For this review, take the finished solid that the model builds, in its own axes (mm). A direction names the side the tool comes from. Round coordinates to 2 decimals unless told otherwise and drop trailing zeros. Order: outer loops, then holes, each group sorted by start corner. A loop starts at its lowest first (then second) coordinate and runs counter-clockwise, first axis right, second up. Notation, with made-up numbers: (50, -31) - (95, -31) arc R8 cw to (95, -21) - close; hole circle Ø3 at (32.5, -19.75). An arc over 180 degrees is marked (long way). One line per question, with ' | ' between items.
```python
from build123d import *

# Parameters (mm, degrees)
SKETCH2_R           = 40
BOSS_EXTRUDE1_DEPTH = 320
SKETCH3_R           = 30
CUT_EXTRUDE1_DEPTH  = 300
CUT_EXTRUDE2_REACH  = 326.962
SKETCH4_R           = 22.5
BOSS_EXTRUDE2_START = 80
SKETCH5_R           = 40
BOSS_EXTRUDE2_DEPTH = 80
SKETCH6_W           = 40
SKETCH6_H           = 78
CUT_EXTRUDE3_DEPTH  = 5
SKETCH7_R           = 15
CUT_EXTRUDE4_DEPTH  = 332.096662623
FILLET2_R           = 5
FILLET3_R           = 2


with BuildPart() as part:
    # Sketch2 → Boss-Extrude1 (new body)
    with BuildSketch(Plane.XY):
        Circle(SKETCH2_R)
    extrude(amount=BOSS_EXTRUDE1_DEPTH)

    # Sketch3 → Cut-Extrude1 (cut)
    with BuildSketch(Plane(origin=(0, 0, 0), x_dir=(-1, 0, 0), z_dir=(0, 0, -1))):
        Circle(SKETCH3_R)
    extrude(amount=-CUT_EXTRUDE1_DEPTH, mode=Mode.SUBTRACT)

    # Sketch4 → Cut-Extrude2 (cut, up to next)
    with BuildSketch(Plane.XY.offset(320), mode=Mode.PRIVATE) as cut_extrude2_sk1:
        Circle(SKETCH4_R)
    cut_extrude2_tool1 = extrude(cut_extrude2_sk1.sketch, amount=-CUT_EXTRUDE2_REACH, mode=Mode.PRIVATE) & part.part
    add(cut_extrude2_tool1.solids().sort_by_distance((0, 0, 320))[0], mode=Mode.SUBTRACT)

    # Sketch5 → Boss-Extrude2 (add)
    with BuildSketch(Plane(origin=(0, 0, 0), x_dir=(-1, 0, 0), z_dir=(0, 0, -1)).offset(BOSS_EXTRUDE2_START)):
        Circle(SKETCH5_R)
    extrude(amount=-BOSS_EXTRUDE2_DEPTH)

    # Sketch6 → Cut-Extrude3 (cut)
    with BuildSketch(Plane(origin=(0, 40, 0), x_dir=(1, 0, 0), z_dir=(0, 1, 0))):
        with Locations((0, 41)):
            Rectangle(SKETCH6_W, SKETCH6_H)
    cut_extrude3 = extrude(amount=-CUT_EXTRUDE3_DEPTH, mode=Mode.SUBTRACT)

    # Mirror1: Cut-Extrude3 across plane
    add(cut_extrude3.mirror(Plane.ZX), mode=Mode.SUBTRACT)

    # Sketch7 → Cut-Extrude4 (cut, through all)
    with BuildSketch(Plane(origin=(0, 35, 0), x_dir=(1, 0, 0), z_dir=(0, 1, 0))):
        with Locations(Location((0, 45, 0), (0, 0, 270))):
            Circle(SKETCH7_R)
    extrude(amount=-CUT_EXTRUDE4_DEPTH, mode=Mode.SUBTRACT)

    # Fillet2
    fillet2_edges = [part.edges().sort_by_distance(p)[0] for p in [
        (40, 0, -80),
        (0, 35, -80),
        (-34.457195687, 20.315060063, -80),
        (0, -35, -80),
        (-40, 0, 320),
    ]]
    fillet(fillet2_edges, radius=FILLET2_R - 0.0001)  # a hair under: the kernel refuses the full size

    # Fillet3
    fillet3_edges = [part.edges().sort_by_distance(p)[0] for p in [
        (0, -35, -60),
        (0, 35, -60),
    ]]
    fillet(fillet3_edges, radius=FILLET3_R)


solid = part.part
```
(1) We need section A-A on x = 0. State the section outline as (y, z) points, plus the area to 3 significant figures.
Output values:
outline: (-40, -2) - (-35, -2) - (-35, -28) arc R2 ccw to (-33, -30) - (33, -30) arc R2 ccw to (35, -28) - (35, -2) - (40, -2) - (40, 315) arc R5 ccw to (35, 320) - (22.5, 320) - (22.5, 300) - (30, 300) - (30, 0) - (-30, 0) - (-30, 300) - (-22.5, 300) - (-22.5, 320) - (-35, 320) arc R5 ccw to (-40, 315) - close; (-35, -75) arc R5 ccw to (-30, -80) - (30, -80) arc R5 ccw to (35, -75) - (35, -62) arc R2 ccw to (33, -60) - (-33, -60) arc R2 ccw to (-35, -62) - close | area: 10,200 mm^2
(2) Insertion check: pin 1 (6 mm diameter, centred on x = 29.5, z = 93.5, fed in from -Y); pin 2 (1.5 mm diameter, centred on y = 24, z = -2.5, fed in from +X); pin 3 (1 mm diameter, centred on x = 19.5, z = 62.5, fed in from -Y). Each pin has a flat end and moves straight along its axis. Give the tip position at first contact, or say it passes through.
Output values:
pin 1: y = -29.96 | pin 2: x = 32.55 | pin 3: y = -35.2
(3) Mouldability with a two-part tool opening along Y and no side actions: class faces 1 (the flat face through (0, 0, 0)), 2 (the flat face through (0, -35, -23)), 3 (the cylindrical face through (29.97, 1.32, 147.9)), 4 (the flat face through (0, 0, -80)) as released by +Y, released by -Y, zero draft, split by the parting line, or undercut.
Output values:
face 1: undercut | face 2: released by -Y | face 3: undercut | face 4: zero draft
(4) We need section B-B on z = -45. State the section outline as (x, y) points, plus the area to 3 significant figures.
Output values:
outline: (-19.36, -35) - (-17, -35) arc R2 ccw to (-15, -33) - (-15, 33) arc R2 ccw to (-17, 35) - (-19.36, 35) arc R40 ccw to start; (15, -33) arc R2 ccw to (17, -35) - (19.36, -35) arc R40 ccw to (19.36, 35) - (17, 35) arc R2 ccw to (15, 33) - close | area: 2,660 mm^2
(5) For probe 1 along X at (y, z) = (19.5, -45); probe 2 along Y at (x, z) = (0, 307); probe 3 along Y at (x, z) = (-17, 214.5), list the stretches that pass through material, from the lowest coordinate up. Write a range as [from, to].
Output values:
probe 1: [-34.92, -15], [15, 34.92] | probe 2: [-40, -22.5], [22.5, 40] | probe 3: [-36.21, -24.72], [24.72, 36.21]
(6) We need section C-C on z = 150. State the section outline as (x, y) points.
Output values:
outline: circle Ø80 at (0, 0); hole circle Ø60 at (0, 0)
(7) For faces 5 (the flat face through (-4.3, 22.4, 300)), 6 (the flat face through (0, 35, -23)), 7 (the cylindrical face through (10.382, -19.961, 310.14)), list the 3-axis set-ups (+Z, -Z, +X, -X, +Y, -Y) from which the entire face can be reached by the end or side of a thin tool; tool diameter is ignored.
Output values:
face 5: none | face 6: -Z, +X, -X, +Y | face 7: +Z
